Build history of the part. All positions in model axes, mm. Face numbers are marked on the shaded views. A direction names the side the tool comes from. Coordinates: 2 decimals unless noted, no trailing zeros. Loops run counter-clockwise (first coordinate to the right, second up) from the corner with the lowest first, then second, coordinate; pieces in that order, holes last. Notation, with made-up numbers: (-7.75, 58.25) - (4.25, 58.25) arc R18 cw to (4.25, 88.25) - close; hole circle Ø9 at (38.5, 68). An arc over 180 degrees is marked (long way). One line per item, written item: value.
```python
from build123d import *

# Parameters (mm, degrees)
SKETCH1_R           = 4.445
BOSS_EXTRUDE1_DEPTH = 1.27
SKETCH2_R           = 3.175
BOSS_EXTRUDE2_DEPTH = 29.21
CUT_EXTRUDE1_START  = -1.5494
SKETCH4_R           = 3.175
SKETCH4_R_2         = 2.921
CUT_EXTRUDE1_DEPTH  = 0.7366
CHAMFER1_SIZE       = 0.254


with BuildPart() as part:
    # Sketch1 → Boss-Extrude1 (new body)
    with BuildSketch(Plane.XY):
        Circle(SKETCH1_R)
    extrude(amount=BOSS_EXTRUDE1_DEPTH)

    # Sketch2 → Boss-Extrude2 (add)
    with BuildSketch(Plane.XY.offset(1.27)):
        with Locations(Location((0, 0, 0), (0, 0, 180))):
            Circle(SKETCH2_R)
    extrude(amount=BOSS_EXTRUDE2_DEPTH)

    # Sketch4 → Cut-Extrude1 (cut)
    with BuildSketch(Plane.XY.offset(30.48).offset(CUT_EXTRUDE1_START)):
        with Locations(Location((0, 0, 0), (0, 0, 180))):
            Circle(SKETCH4_R)
        Circle(SKETCH4_R_2, mode=Mode.SUBTRACT)
    extrude(amount=CUT_EXTRUDE1_DEPTH, mode=Mode.SUBTRACT)

    # Chamfer1
    chamfer1_edges = [part.edges().sort_by_distance(p)[0] for p in [
        (3.175, 0, 30.48),
    ]]
    chamfer(chamfer1_edges, length=CHAMFER1_SIZE)


solid = part.part
```
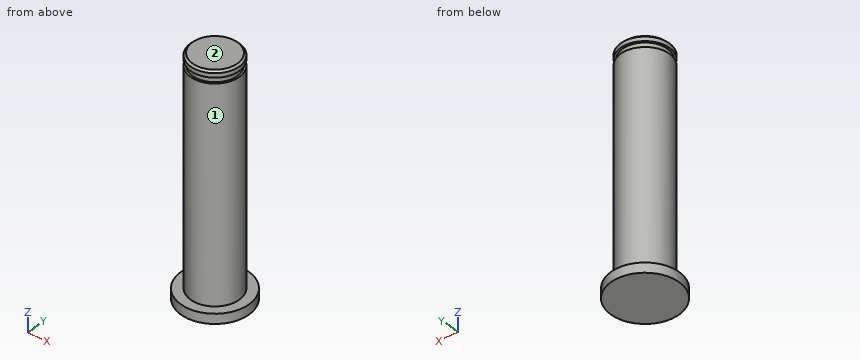
Item 1: Probe probe 1 along Z at (x, y) = (-3.75, 1.75); probe 2 along Z at (x, y) = (2.5, -1.75); probe 3 along Y at (x, z) = (0, 6) (3 decimals). List the from-to ranges inside material, lowest first. Write a range as from..to.
Check result:
probe 1: z = 0..1.27
probe 2: z = 0..28.93, 29.67..30.35
probe 3: y = -3.175..3.175
Item 2: Tool access for the marked faces 1 and 2: list every direction of +Z, -Z, +X, -X, +Y, -Y with a clear straight run to the whole face (end or side of a thin tool).
Check result:
face 1: +Z
face 2: +Z, +X, -X, +Y, -Y
Item 3: Cut at C-C, the plane z = 18. Write the cut outline in (x, y) (3 decimals), then the cut area to 3 significant figures.
Check result:
outline: circle Ø6.35 at (0, 0)
area: 31.7 mm^2
Item 4: Drop flat-ended pins along their axis: P1, Ø1, axis at y = -1, z = 11.5, coming from the -X side; P2, Ø4, axis at x = 3.5, z = 17, coming from the -Y side; P3, Ø2, axis at x = 1, z = 27, coming from the +Y side (3 decimals). Give the stop position or say it passes through.
Check result:
P1: stops at x = -3.14
P2: stops at y = -2.8
P3: stops at y = 3.175
Item 5: Cut at D-D, the plane y = 4. Write the cut outline in (x, z).
Check result:
outline: (-1.94, 0) - (1.94, 0) - (1.94, 1.27) - (-1.94, 1.27) - close
Item 6: Cut at A-A, the plane y = 0. Write the cut outline in (x, z) (3 decimals), then the cut area to 3 significant figures.
Check result:
outline: (-4.445, 0) - (4.445, 0) - (4.445, 1.27) - (3.175, 1.27) - (3.175, 28.931) - (2.921, 28.931) - (2.921, 29.667) - (3.175, 29.667) - (3.175, 30.226) - (2.921, 30.48) - (-2.921, 30.48) - (-3.175, 30.226) - (-3.175, 29.667) - (-2.921, 29.667) - (-2.921, 28.931) - (-3.175, 28.931) - (-3.175, 1.27) - (-4.445, 1.27) - close
area: 196 mm^2
